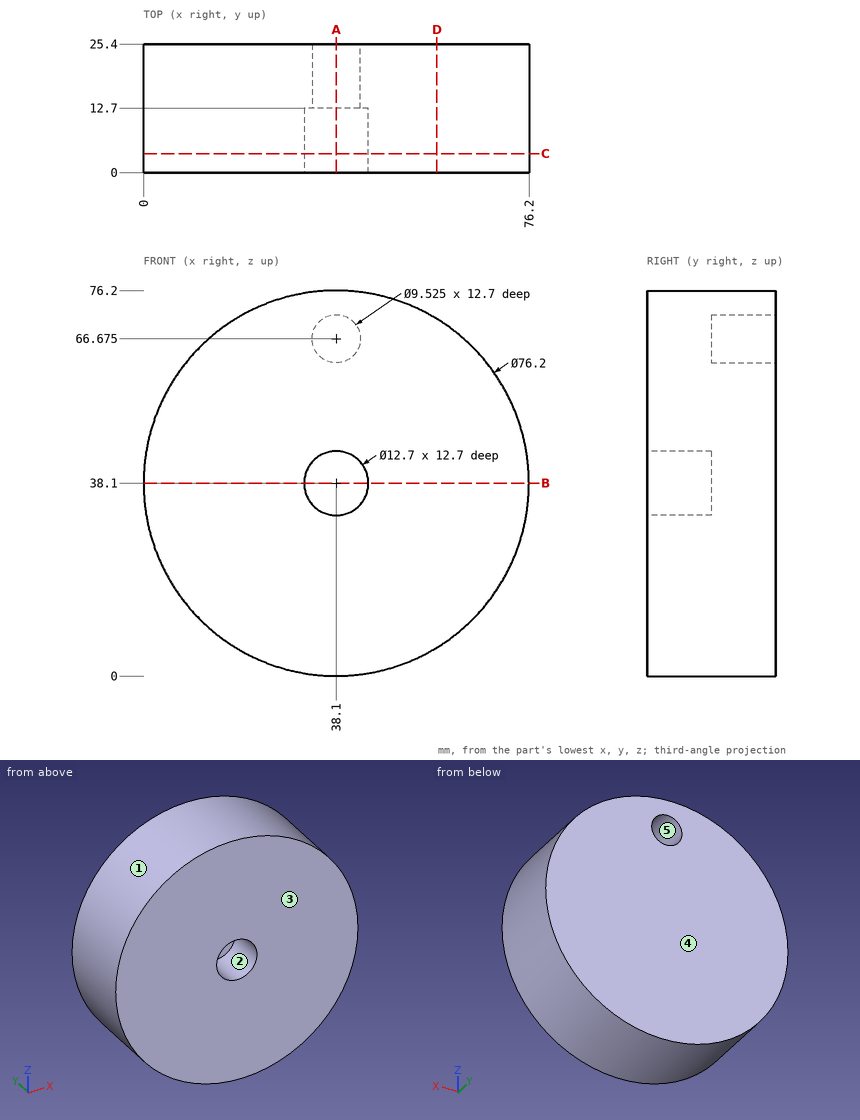
Geometry check sheet. Reference: drawing and pictorial views, mm from the part's lowest x, y, z. A direction names the side the tool comes from. Round coordinates to 2 decimals unless told otherwise and drop trailing zeros. Order: outer loops, then holes, each group sorted by start corner. A loop starts at its lowest first (then second) coordinate and runs counter-clockwise, first axis right, second up. Notation, with made-up numbers: (-28, 62.25) - (-11, 62.25) arc R36 cw to (-11, 97.25) - close; hole circle Ø6 at (-4, 53.5). An arc over 180 degrees is marked (long way). Write item = value, one per line.
Q1. Section check A-A (x = 38.1). Record the boundary of the cut face in (y, z), and give its area (3 significant figures).
Computed:
outline = (0, 0) - (25.4, 0) - (25.4, 61.91) - (12.7, 61.91) - (12.7, 71.44) - (25.4, 71.44) - (25.4, 76.2) - (0, 76.2) - (0, 44.45) - (12.7, 44.45) - (12.7, 31.75) - (0, 31.75) - close
area = 1,650 mm^2
Q2. Go/stop test with flat-tipped pins: pin 1 (5 mm diameter, centred on x = 35.5, y = 18, fed in from +Z); pin 2 (1.5 mm diameter, centred on x = 36.5, z = 10.5, fed in from -Y); pin 3 (3 mm diameter, centred on x = 28.5, y = 11.5, fed in from -Z); pin 4 (3 mm diameter, centred on x = 42, y = 6.5, fed in from +Z). Record where each tip stops, or that it passes through.
Computed:
pin_1 = 76.2
pin_2 = 0
pin_3 = 0.87
pin_4 = 76.12
Q3. Section check C-C (y = 3.75). Record the boundary of the cut face in (x, z).
Computed:
outline = circle Ø76.2 at (38.1, 38.1); hole circle Ø12.7 at (38.1, 38.1)
Q4. Tool access check on the marked faces 4 and 5. Record the directions out of +Z, -Z, +X, -X, +Y, -Y that give a thin tool (end or side, any length) a straight path to the whole face; none if there is none.
Computed:
face_4 = +Z, -Z, +X, -X, +Y
face_5 = +Y
Q5. Section check D-D (x = 58). Record the boundary of the cut face in (y, z).
Computed:
outline = (0, 5.61) - (25.4, 5.61) - (25.4, 70.59) - (0, 70.59) - close
Q6. Draft check along X on the marked faces 1, 2 and 3. Enter one of: pulls with the +X half, pulls with the -X half, needs draft (parallel to the pull), parting line crosses it, or undercut.
Computed:
face_1 = parting line crosses it
face_2 = undercut
face_3 = needs draft
Q7. Section check B-B (z = 38.1). Record the boundary of the cut face in (x, y).
Computed:
outline = (0, 0) - (31.75, 0) - (31.75, 12.7) - (44.45, 12.7) - (44.45, 0) - (76.2, 0) - (76.2, 25.4) - (0, 25.4) - close
Q8. Thickness scan on line 1 along Z through (x, y) = (38.1, 19.25); line 2 along Z through (x, y) = (38.1, 9.5); line 3 along X through (y, z) = (15.75, 65). Record the ranges inside material, lowest first.
Computed:
line_1 = 0 to 61.91, 71.44 to 76.2
line_2 = 0 to 31.75, 44.45 to 76.2
line_3 = 11.12 to 33.64, 42.56 to 65.08
